CAD build for the part. Positions are in the model's coordinates, mm. A direction names the side the tool comes from. Round coordinates to 2 decimals unless told otherwise and drop trailing zeros. Order: outer loops, then holes, each group sorted by start corner. A loop starts at its lowest first (then second) coordinate and runs counter-clockwise, first axis right, second up. Notation, with made-up numbers: (28.25, -10.5) - (84.25, -10.5) arc R23 cw to (84.25, 1.5) - close; hole circle Ø7 at (3, 15). An arc over 180 degrees is marked (long way). Use one line per item in the form item = value. Start each with the question number.
from build123d import *

# Parameters (mm, degrees)
BOSS_EXTRUDE1_DEPTH = 10.922
CUT_EXTRUDE1_DEPTH  = 114.427
SKETCH4_R           = 1.778
CUT_EXTRUDE2_DEPTH  = 114.427
SKETCH5_R           = 1.778
CUT_EXTRUDE3_DEPTH  = 114.427
SKETCH6_R           = 1.778
CUT_EXTRUDE4_DEPTH  = 251.079
FILLET1_R           = 2.54
FILLET2_R           = 2.54
FILLET3_R           = 2.54
FILLET4_R           = 2.54
FILLET5_R           = 2.54
FILLET6_R           = 2.54


with BuildPart() as part:
    # Sketch1 → Boss-Extrude1 (new body)
    with BuildSketch(Plane.XY):
        Polygon((0, -25.411879188), (0, 0), (-6.985, 0), (-6.985, -25.411879188), (27.675318213, -85.445311339), (-114.035318213, -85.445311339), (-79.375, -25.411879188), (-79.375, 0), (-86.36, 0), (-86.36, -25.411879188), (-137.955366837, -114.777675985), (-137.955366837, -126.876050876), (-130.713866793, -126.876050876), (-130.713866793, -114.333404876), (-116.677285334, -90.021332625), (30.317285334, -90.021332625), (44.353866793, -114.333404876), (44.353866793, -126.876050876), (51.595366837, -126.876050876), (51.595366837, -114.777675985), align=None)
    extrude(amount=BOSS_EXTRUDE1_DEPTH)

    # Sketch3 → Cut-Extrude1 (cut)
    with BuildSketch(Plane(origin=(0, 0, 0), x_dir=(0, 0, -1), z_dir=(1, 0, 0))):
        Polygon((-2.471808629, 0), (-2.492726697, 0), (-8.450191371, 0), (-8.450191371, -8.061399091), (-5.461, -12.079224104), (-2.471808629, -8.061399091), align=None)
    extrude(amount=-CUT_EXTRUDE1_DEPTH, mode=Mode.SUBTRACT)

    # Sketch4 → Cut-Extrude2 (cut)
    with BuildSketch(Plane.XY.offset(10.922)):
        with Locations((-3.4925, -3.83202166)):
            Circle(SKETCH4_R)
    extrude(amount=-CUT_EXTRUDE2_DEPTH, mode=Mode.SUBTRACT)

    # Sketch5 → Cut-Extrude3 (cut)
    with BuildSketch(Plane.XY.offset(10.922)):
        with Locations((-82.8675, -3.918997874)):
            Circle(SKETCH5_R)
    extrude(amount=-CUT_EXTRUDE3_DEPTH, mode=Mode.SUBTRACT)

    # Sketch6 → Cut-Extrude4 (cut)
    with BuildSketch(Plane(origin=(51.595366837, 0, 0), x_dir=(0, 0, -1), z_dir=(1, 0, 0))):
        with Locations((-5.461, -120.687777383)):
            Circle(SKETCH6_R)
    extrude(amount=-CUT_EXTRUDE4_DEPTH, mode=Mode.SUBTRACT)

    # Fillet1
    fillet1_edges = [part.edges().sort_by_distance(p)[0] for p in [
        (37.335576064, -102.177368751, 10.922),
        (25.797683419, -70.094777586, 10.922),
        (10.345159107, -55.428595263, 10.922),
    ]]
    fillet(fillet1_edges, radius=FILLET1_R)

    # Fillet2
    fillet2_edges = [part.edges().sort_by_distance(p)[0] for p in [
        (10.345159107, -55.428595263, 0),
        (25.797683419, -70.094777586, 0),
        (37.335576064, -102.177368751, 0),
    ]]
    fillet(fillet2_edges, radius=FILLET2_R)

    # Fillet3
    fillet3_edges = [part.edges().sort_by_distance(p)[0] for p in [
        (-41.713530316, -85.445311339, 10.922),
    ]]
    fillet(fillet3_edges, radius=FILLET3_R)

    # Fillet4
    fillet4_edges = [part.edges().sort_by_distance(p)[0] for p in [
        (-41.713530316, -85.445311339, 0),
    ]]
    fillet(fillet4_edges, radius=FILLET4_R)

    # Fillet5
    fillet5_edges = [part.edges().sort_by_distance(p)[0] for p in [
        (-97.438393948, -56.698595263, 0),
        (-123.695576064, -102.177368751, 10.922),
        (-112.157683419, -70.094777586, 10.922),
        (-97.438393948, -56.698595263, 10.922),
    ]]
    fillet(fillet5_edges, radius=FILLET5_R)

    # Fillet6
    fillet6_edges = [part.edges().sort_by_distance(p)[0] for p in [
        (-112.157683419, -70.094777586, 0),
        (-123.695576064, -102.177368751, 0),
    ]]
    fillet(fillet6_edges, radius=FILLET6_R)


solid = part.part
(1) Flat gauge pins, fed straight in: P1, Ø3.5, axis at y = -11.5, z = 7, coming from the -X side; P2, Ø4.5, axis at y = -120.69, z = 5.46, coming from the -X side; P3, Ø5.5, axis at y = -17, z = 7.5, coming from the +X side; P4, Ø1, axis at x = 21.5, z = 8.5, coming from the -Y side. Where does each tip first touch, or does it go through?
(2) Which spindle directions (+Z, -Z, +X, -X, +Y, -Y) get a long thin tool onto all of the face, cutting with end or side? Do faces 4 (the cylindrical face through (-124.225, -101.645, 10.158)), 5 (the cylindrical face through (-97.61, -55.54, 10.16)), 6 (the flat face through (-3, -6, 2.472)). Say none if no direction does.
(3) Slice it at A-A (x = -50). Give the cut face in (y, z), and give its area (3 significant figures).
(4) Wall check: line 1 (X direction, y = -118, z = 0.5); line 2 (X direction, y = -18, z = 3) (3 decimals); line 3 (Y direction, x = -50, z = 3.5). Give the ranges that are in metal, low to high. Write a range as [from, to].
(5) Mould opens along Y. For faces 1 (the flat face through (-137.955, -122, 7)), 2 (the cylindrical face through (48.025, -118.925, 5.692)), 3 (the flat face through (-123.794, -102.348, 5.42)) say: pulls with the +Y half, pulls with the -Y half, needs draft (parallel to the pull), parting line crosses it, or undercut.
Results list:
q1.P1 = -86.36
q1.P2 = -137.96
q1.P3 = 0
q1.P4 = -90.02
q2.face_4 = +Z, -Y
q2.face_5 = +Z
q2.face_6 = +X, -X, +Y
q3.outline = (-90.02, 0) - (-87.99, 0) arc R2.54 ccw to (-85.45, 2.54) - (-85.45, 8.38) arc R2.54 ccw to (-87.99, 10.92) - (-90.02, 10.92) - close
q3.area = 47.2 mm²
q4.line_1 = [-137.96, -130.71], [44.35, 51.6]
q4.line_2 = [-86.36, -79.375], [-6.985, 0]
q4.line_3 = [-90.02, -85.45]
q5.face_1 = needs draft
q5.face_2 = undercut
q5.face_3 = pulls with the -Y half
